```python
from build123d import *

# Parameters (mm, degrees)
SKETCH_1_W      = 90
SKETCH_1_H      = 55
SKETCH_1_R      = 1.25
EXTRUDE_1_DEPTH = 3
SKETCH_2_R      = 3
EXTRUDE_2_DEPTH = 3
SKETCH_3_W      = 15
SKETCH_3_H      = 10
SKETCH_3_R      = 3
EXTRUDE_3_DEPTH = 4
CHAMFER_1_SIZE  = 1
SKETCH_4_R      = 2.5
SKETCH_4_R_2    = 1.25
EXTRUDE_4_DEPTH = 2
FILLET_1_R      = 4


with BuildPart() as part:
    # Эскиз1 → Бобышка-Вытянуть1 (new body)
    with BuildSketch(Plane.XY):
        with Locations((45, 27.5)):
            Rectangle(SKETCH_1_W, SKETCH_1_H)
        with Locations((6, 31)):
            Circle(SKETCH_1_R, mode=Mode.SUBTRACT)
        with Locations((6, 6)):
            Circle(SKETCH_1_R, mode=Mode.SUBTRACT)
        with Locations((53, 39)):
            Circle(SKETCH_1_R, mode=Mode.SUBTRACT)
        with Locations((53, 6)):
            Circle(SKETCH_1_R, mode=Mode.SUBTRACT)
        with Locations((63, 6)):
            Circle(SKETCH_1_R, mode=Mode.SUBTRACT)
        with Locations((63, 52)):
            Circle(SKETCH_1_R, mode=Mode.SUBTRACT)
        with Locations((84, 52)):
            Circle(SKETCH_1_R, mode=Mode.SUBTRACT)
        with Locations((84, 6)):
            Circle(SKETCH_1_R, mode=Mode.SUBTRACT)
    extrude(amount=EXTRUDE_1_DEPTH)

    # Эскиз2 → Бобышка-Вытянуть2 (add)
    with BuildSketch(Plane.XY.offset(3)):
        with BuildLine():
            Line((0, 55), (-15, 55))
            Line((-15, 55), (-15, 45))
            Line((-15, 45), (-4, 45))
            ThreePointArc((-4, 45), (-1.171572875, 43.828427125), (0, 41))
            Line((0, 41), (0, 55))
        make_face()
        with BuildLine():
            Line((0, 0), (-6, 0))
            ThreePointArc((-6, 0), (-12, 6), (-6, 12))
            Line((-6, 12), (-4, 12))
            ThreePointArc((-4, 12), (-1.171572875, 13.171572875), (0, 16))
            Line((0, 16), (0, 0))
        make_face()
        with Locations((-6, 6)):
            Circle(SKETCH_2_R, mode=Mode.SUBTRACT)
        with BuildLine():
            Line((90, 55), (96, 55))
            ThreePointArc((96, 55), (102, 49), (96, 43))
            Line((96, 43), (94, 43))
            ThreePointArc((94, 43), (91.171572875, 41.828427125), (90, 39))
            Line((90, 39), (90, 55))
        make_face()
        with Locations((96, 49)):
            Circle(SKETCH_2_R, mode=Mode.SUBTRACT)
    extrude(amount=-EXTRUDE_2_DEPTH)

    # Эскиз3 → Бобышка-Вытянуть3 (add)
    with BuildSketch(Plane(origin=(0, 55, 0), x_dir=(1, 0, 0), z_dir=(0, 1, 0))):
        with Locations((-7.5, -8)):
            Rectangle(SKETCH_3_W, SKETCH_3_H)
        with Locations((-7.5, -8.5)):
            Circle(SKETCH_3_R, mode=Mode.SUBTRACT)
    extrude(amount=-EXTRUDE_3_DEPTH)

    # Фаска1
    chamfer_1_edges = [part.edges().sort_by_distance(p)[0] for p in [
        (-7.5, 51, 3),
        (0, 53, 3),
    ]]
    chamfer(chamfer_1_edges, length=CHAMFER_1_SIZE)

    # Эскиз4 → Бобышка-Вытянуть4 (add)
    with BuildSketch(Plane.XY.offset(3)):
        with Locations((63, 52)):
            Circle(SKETCH_4_R)
        with Locations((63, 52)):
            Circle(SKETCH_4_R_2, mode=Mode.SUBTRACT)
        with Locations((84, 52)):
            Circle(SKETCH_4_R)
        with Locations((84, 52)):
            Circle(SKETCH_4_R_2, mode=Mode.SUBTRACT)
        with Locations((63, 6)):
            Circle(SKETCH_4_R)
        with Locations((63, 6)):
            Circle(SKETCH_4_R_2, mode=Mode.SUBTRACT)
        with Locations((84, 6)):
            Circle(SKETCH_4_R)
        with Locations((84, 6)):
            Circle(SKETCH_4_R_2, mode=Mode.SUBTRACT)
    extrude(amount=EXTRUDE_4_DEPTH)

    # Скругление1
    fillet_1_edges = [part.edges().sort_by_distance(p)[0] for p in [
        (-15, 45, 1.5),
        (90, 0, 1.5),
        (-15, 53, 13),
        (0, 53, 13),
    ]]
    fillet(fillet_1_edges, radius=FILLET_1_R)


solid = part.part
```
The model under review builds one solid part; all positions refer to its coordinate system, in mm. A direction names the side the tool comes from. Round coordinates to 2 decimals unless told otherwise and drop trailing zeros. Loops run counter-clockwise (first coordinate to the right, second up) from the corner with the lowest first, then second, coordinate; pieces in that order, holes last. Notation, with made-up numbers: (-25.75, 1) - (-8.75, 1) arc R27 cw to (-8.75, 29) - close; hole circle Ø5 at (-33, 63). An arc over 180 degrees is marked (long way). Write each question's results on one line, items separated by ' | '. Start each with the question number.
Q1. Take a section at A-A on x = 53. Give the boundary of the cut face in (y, z).
Q2. Take a section at C-C on z = 7.25. Give the boundary of the cut face in (x, y), plus the area to 3 significant figures.
Q3. Take a section at B-B on x = -7.5. Give the boundary of the cut face in (y, z), plus the area to 3 significant figures.
Q4. Insertion check: P1, Ø1.5, axis at x = 83, y = 6.5, coming from the +Z side; P2, Ø3.5, axis at x = -9, z = 1.5, coming from the -Y side; P3, Ø0.9, axis at y = 29.5, z = 1, coming from the -X side. Each pin has a flat end and moves straight along its axis. Give the tip position at first contact, or say it passes through.
Q5. Wall thickness on line 1 along Y through (x, z) = (53, 2.4); line 2 along Y through (x, z) = (6, 1.95); line 3 along Y through (x, z) = (96, 0.95): over which ranges is each line inside the solid? List them lowest first. Write a range as [from, to].
Q6. Draft analysis for pull direction X (two halves, no side actions). For faces 4 (the cylindrical face through (81.5, 6.1, 4)), 5 (the flat face through (-8, 51, 5)), 6 (the cylindrical face through (-13.797, 46.141, 1.479)), state which applies: pulls with the +X half, pulls with the -X half, needs draft (parallel to the pull), parting line crosses it, or undercut.
Q7. Take a section at D-D on y = 35. Give the boundary of the cut face in (x, z), plus the area to 3 significant figures.
Q8. Tool access review of faces 1 (the cylindrical face through (65.385, 6.751, 3.986)), 2 (the flat face through (95, 43, 2)), 3 (the cylindrical face through (-1.203, 43.859, 1.521)): name each direction out of +Z, -Z, +X, -X, +Y, -Y from which nothing blocks a thin tool from reaching the whole face with its end or side.
Data:
1) outline: (0, 0) - (4.75, 0) - (4.75, 3) - (0, 3) - close; (7.25, 0) - (37.75, 0) - (37.75, 3) - (7.25, 3) - close; (40.25, 0) - (55, 0) - (55, 3) - (40.25, 3) - close
2) outline: (-15, 51) - (-10.23, 51) - (-10.23, 55) - (-15, 55) - close; (-4.77, 51) - (0, 51) - (0, 55) - (-4.77, 55) - close | area: 38.2 mm²
3) outline: (0.19, 0) - (3.4, 0) - (3.4, 3) - (0.19, 3) - close; (8.6, 0) - (11.81, 0) - (11.81, 3) - (8.6, 3) - close; (45, 0) - (55, 0) - (55, 5.5) - (51, 5.5) - (51, 4) - (50, 3) - (45, 3) - close; (51, 11.5) - (55, 11.5) - (55, 13) - (51, 13) - close | area: 65.8 mm²
4) P1: stops at z = 5 | P2: stops at y = 0.13 | P3: stops at x = 0
5) line 1: y = [0, 4.75], [7.25, 37.75], [40.25, 55] | line 2: y = [0, 4.75], [7.25, 29.75], [32.25, 55] | line 3: y = [43, 46], [52, 55]
6) face 4: undercut | face 5: needs draft | face 6: pulls with the -X half
7) outline: (0, 0) - (90, 0) - (90, 3) - (0, 3) - close | area: 270 mm²
8) face 1: +Z | face 2: +Z, -Z, +X, -Y | face 3: +Z, -Z, -X
